Check sheet for the modelled part. Datum: model origin and axes. Units: mm. Give positions to 0.01 mm unless a question says otherwise; leave off trailing zeros.
Item 1: Material ranges on line 1 along Y through (x, z) = (36, 30.5); line 2 along X through (y, z) = (3, -4), recorded low to high.
Item 2: Sectioned sample at A-A on y = 23. Count the separate pieces of the cut face and the enclosed holes in it, and give its area (3 significant figures).
Item 3: Gauge pin test, flat ends, axial feed: P1, Ø0.5, axis at x = 20.5, z = -9.5, coming from the +Y side; P2, Ø1.5, axis at y = 14.5, z = 23.5, coming from the +X side; P3, Ø3, axis at y = 5.5, z = 31.5, coming from the -X side. Record the tip position at first contact, or that the pin passes through.
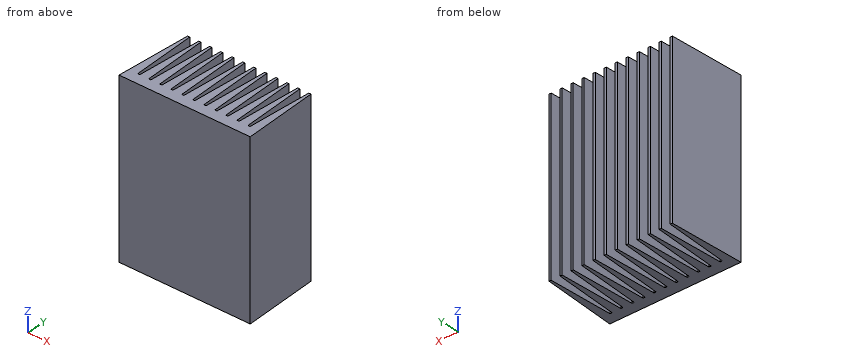
from build123d import *

# Parameters (mm, degrees)
BOSS_EXTRUDE1_DEPTH = 39.5


with BuildPart() as part:
    # Sketch1 → Boss-Extrude1 (new, symmetric)
    with BuildSketch(Plane.XY):
        Polygon((0, 0), (1.834272275, 35), (2.834272275, 35), (4.406505653, 5), (5.406505653, 5), (6.978739032, 35), (7.978739032, 35), (9.55097241, 5), (10.55097241, 5), (12.123205789, 35), (13.123205789, 35), (14.695439167, 5), (15.695439167, 5), (17.267672546, 35), (18.267672546, 35), (19.839905924, 5), (20.839905924, 5), (22.412139303, 35), (23.412139303, 35), (24.984372681, 5), (25.984372681, 5), (27.55660606, 35), (28.55660606, 35), (30.128839438, 5), (31.128839438, 5), (32.701072817, 35), (33.701072817, 35), (35.273306195, 5), (36.273306195, 5), (37.845539574, 35), (38.845539574, 35), (40.417772952, 5), (41.417772952, 5), (42.990006331, 35), (43.990006331, 35), (45.562239709, 5), (46.562239709, 5), (48.134473088, 35), (49.134473088, 35), (50.706706466, 5), (51.706706466, 5), (53.278939845, 35), (54.278939845, 35), (55.851173223, 5), (56.851173223, 5), (58.423406602, 35), (59.423406602, 35), (61.257678877, 0), align=None)
    extrude(amount=BOSS_EXTRUDE1_DEPTH, both=True)


solid = part.part
Report:
1. line 1: y = 0 to 5
1. line 2: x = 0.16 to 61.1
2. separate pieces: 12
2. enclosed holes: 0
2. area: 2,140 mm2
3. P1: stops at y = 5
3. P2: stops at x = 60.54
3. P3: stops at x = 0.21
